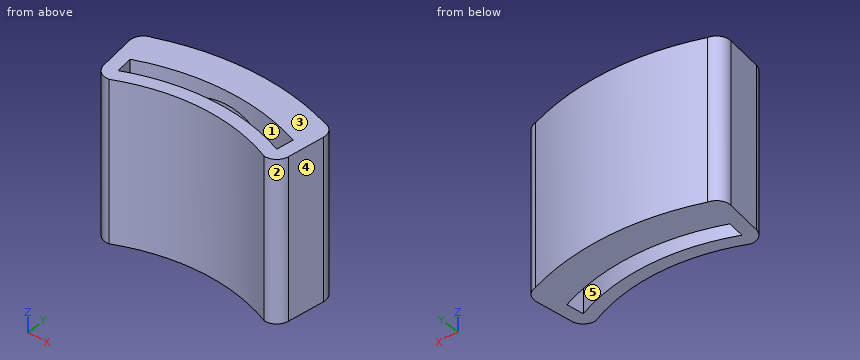
from build123d import *

# Parameters (mm, degrees)
BOSS_EXTRUDE1_DEPTH                 = 24
BOSS_EXTRUDE1_2_DEPTH               = 24
SKETCH4_R                           = 10
CUT_EXTRUDE1_DEPTH                  = 2.5
CUT_EXTRUDE1_DIRECTION_2_REACH      = 30.177
CUT_EXTRUDE1_DIRECTION_2_END_RADIUS = 32.507235283
SKETCH5_W                           = 24
SKETCH5_H                           = 9.578050903
BOSS_EXTRUDE2_DEPTH                 = 2
SKETCH6_W                           = 24
SKETCH6_H                           = 9.578050903
BOSS_EXTRUDE3_DEPTH                 = 2
FILLET1_R                           = 2


with BuildPart() as part:
    # Sketch1 → Boss-Extrude1 (new body)
    with BuildSketch(Plane.XY):
        with BuildLine():
            Line((-13, 35.007235283), (-12.343096138, 30.072717261))
            ThreePointArc((-12.343096138, 30.072717261), (0, 32.507235283), (12.343096138, 30.072717261))
            Line((12.343096138, 30.072717261), (13, 35.007235283))
            ThreePointArc((13, 35.007235283), (0, 37.343092027), (-13, 35.007235283))
        make_face()
    extrude(amount=BOSS_EXTRUDE1_DEPTH)

    # Sketch4 → Cut-Extrude1 (cut)
    with BuildSketch(Plane(origin=(0, 32.51, 0), x_dir=(1, 0, 0), z_dir=(0, 1, 0))):
        with Locations(Location((0, -12, 0), (0, 0, 270))):
            Circle(SKETCH4_R)
    extrude(amount=CUT_EXTRUDE1_DEPTH, mode=Mode.SUBTRACT)

    # Cut-Extrude1 direction 2: up to this cylinder (the profile starts outside it)
    cut_extrude1_direction_2_end = Plane(origin=(0, 0, 12), z_dir=(0, 0, -1)) * Cylinder(CUT_EXTRUDE1_DIRECTION_2_END_RADIUS, 126.368470565, mode=Mode.PRIVATE)
    # Sketch4 → Cut-Extrude1 direction 2 (cut, up to the surface)
    with BuildSketch(Plane(origin=(0, 32.51, 0), x_dir=(1, 0, 0), z_dir=(0, 1, 0)), mode=Mode.PRIVATE) as cut_extrude1_direction_2_sk1:
        with Locations(Location((0, -12, 0), (0, 0, 270))):
            Circle(SKETCH4_R)
    cut_extrude1_direction_2_tool1 = extrude(cut_extrude1_direction_2_sk1.sketch, amount=-CUT_EXTRUDE1_DIRECTION_2_REACH, mode=Mode.PRIVATE) - cut_extrude1_direction_2_end
    add(cut_extrude1_direction_2_tool1.solids().sort_by_distance((0, 32.51, 12))[0], mode=Mode.SUBTRACT)



with BuildPart() as body_2:
    # Sketch1 → Boss-Extrude1 2 (new body)
    with BuildSketch(Plane.XY):
        with BuildLine():
            Line((11.736079894, 25.5129441), (12, 27.49545417))
            ThreePointArc((12, 27.49545417), (0, 30), (-12, 27.49545417))
            Line((-12, 27.49545417), (-11.736079894, 25.5129441))
            ThreePointArc((-11.736079894, 25.5129441), (0, 28.082839741), (11.736079894, 25.5129441))
        make_face()
    extrude(amount=BOSS_EXTRUDE1_2_DEPTH)


with BuildPart() as part_1:
    add(part.part)

    add(body_2.part)  # Boss-Extrude2 merges body 2
    # Sketch5 → Boss-Extrude2 (add)
    with BuildSketch(Plane(origin=(-8.194466309, -1.090881934, 0), x_dir=(0, 0, 1), z_dir=(-0.9912550349784054, -0.13196005315988815, 0))):
        with Locations((12, 31.627553475)):
            Rectangle(SKETCH5_W, SKETCH5_H)
    extrude(amount=BOSS_EXTRUDE2_DEPTH)

    # Sketch6 → Boss-Extrude3 (add)
    with BuildSketch(Plane(origin=(8.194466309, -1.090881934, 0), x_dir=(0, 0, -1), z_dir=(0.9912550349784054, -0.13196005315988815, 0))):
        with Locations((-12, 31.627553475)):
            Rectangle(SKETCH6_W, SKETCH6_H)
    extrude(amount=BOSS_EXTRUDE3_DEPTH)

    # Fillet1
    fillet1_edges = [part_1.edges().sort_by_distance(p)[0] for p in [
        (-14.98251007, 34.743315176, 12),
        (-13.718589964, 25.249023993, 12),
        (13.718589964, 25.249023993, 12),
        (14.98251007, 34.743315176, 12),
    ]]
    fillet(fillet1_edges, radius=FILLET1_R - 0.0001)  # a hair under: the kernel refuses the full size


solid = part_1.part
Design review of the part built by this model. Coordinates are the model's own, in mm. Face numbers are marked on the shaded views. A direction names the side the tool comes from. Round coordinates to 2 decimals unless told otherwise and drop trailing zeros. Write each loop counter-clockwise with the first axis right and the second up, starting at its lowest first coordinate (ties: lowest second). Pieces come first, ordered by that corner, then holes. Notation, with made-up numbers: (47.25, 1) - (65.25, 1) arc R17 ccw to (65.25, 5) - close; hole circle Ø10 at (11.5, -22.75). An arc over 180 degrees is marked (long way). Return JSON: item names as keys, results as strings. Group by question number.
Item 1: We need section C-C on y = 31.25. Write out the cut boundary in (x, z).
Item 2: We need section A-A on x = 0. Write out the cut boundary in (y, z).
Item 3: The part is to be moulded in two halves that separate along Y. For the marked faces 1, 2 and 3, say which applies: pulls with the +Y half, pulls with the -Y half, needs draft (parallel to the pull), parting line crosses it, or undercut.
Item 4: We need section D-D on y = 33.5. Write out the cut boundary in (x, z), and give its area (3 significant figures).
Item 5: For probe 1 along Y at (x, z) = (-0.25, 1.5); probe 2 along Y at (x, z) = (0.5, 5.75); probe 3 along Z at (x, y) = (-6.25, 33.75), list the stretches that pass through material, from the lowest coordinate up. Write a range as [from, to].
Item 6: Insertion check: P1, Ø8, axis at x = 7, z = 8.5, coming from the -Y side; P2, Ø12, axis at x = 0, z = 12, coming from the -Y side; P3, Ø10, axis at x = -2, z = 7, coming from the -Y side. Each pin has a flat end and moves straight along its axis. Give the tip position at first contact, or say it passes through.
Item 7: Machinability: for the marked faces 4 and 5, which of the approach directions +Z, -Z, +X, -X, +Y, -Y give a long, thin tool a straight path to every point of the face, cutting with its end or side? Answer none if there is none.
Model answer:
{
 "1": {"outline": "(-14.52, 0) - (-8.95, 0) - (-8.95, 7.55) arc R10 cw to (-8.95, 16.45) - (-8.95, 24) - (-14.52, 24) - close; (8.95, 0) - (14.52, 0) - (14.52, 24) - (8.95, 24) - (8.95, 16.45) arc R10 cw to (8.95, 7.55) - close"},
 "2": {"outline": "(28.08, 0) - (30, 0) - (30, 24) - (28.08, 24) - close; (32.51, 0) - (37.34, 0) - (37.34, 24) - (32.51, 24) - (32.51, 22) - (35.01, 22) - (35.01, 2) - (32.51, 2) - close"},
 "3": {"face 1": "undercut", "face 2": "pulls with the -Y half", "face 3": "needs draft"},
 "4": {"outline": "(-14.68, 0) - (14.68, 0) - (14.68, 24) - (-14.68, 24) - close; hole circle Ø20 at (0, 12)", "area": "390 mm²"},
 "5": {"probe 1": "y = [28.08, 30], [32.51, 37.34]", "probe 2": "y = [28.08, 30], [35.01, 37.34]", "probe 3": "z = [0, 4.19], [19.81, 24]"},
 "6": {"P1": "stops at y = 25.84", "P2": "stops at y = 27.43", "P3": "stops at y = 27.2"},
 "7": {"face 4": "+Z, -Z, +X, -Y", "face 5": "+Z, -Z"}
}
